from build123d import *

# Parameters (mm, degrees)
EXTRUDE_THIN1_DEPTH         = 393.7
F_1_4_CLEARANCE_HOLE1_D     = 6.7564
F_1_4_CLEARANCE_HOLE2_D     = 6.7564
F_1_4_CLEARANCE_HOLE2_DEPTH = 1.4478
CUT_EXTRUDE1_DEPTH          = 9.525


with BuildPart() as part:
    # Sketch1 → Extrude-Thin1 (new, symmetric)
    with BuildSketch(Plane(origin=(0, 0, 0), x_dir=(0, 0, -1), z_dir=(1, 0, 0))):
        with BuildLine():
            Line((-10.16, 25.4), (10.16, 25.4))
            ThreePointArc((10.16, 25.4), (11.956051224, 24.656051224), (12.7, 22.86))
            Line((12.7, 22.86), (12.7, -22.86))
            ThreePointArc((12.7, -22.86), (11.956051224, -24.656051224), (10.16, -25.4))
            Line((10.16, -25.4), (-10.16, -25.4))
            ThreePointArc((-10.16, -25.4), (-11.956051224, -24.656051224), (-12.7, -22.86))
            Line((-12.7, -22.86), (-12.7, 22.86))
            ThreePointArc((-12.7, 22.86), (-11.956051224, 24.656051224), (-10.16, 25.4))
        make_face()
        with BuildLine():
            Line((-10.16, 23.9522), (10.16, 23.9522))
            ThreePointArc((10.16, 23.9522), (10.932302026, 23.632302026), (11.2522, 22.86))
            Line((11.2522, 22.86), (11.2522, -22.86))
            ThreePointArc((11.2522, -22.86), (10.932302026, -23.632302026), (10.16, -23.9522))
            Line((10.16, -23.9522), (-10.16, -23.9522))
            ThreePointArc((-10.16, -23.9522), (-10.932302026, -23.632302026), (-11.2522, -22.86))
            Line((-11.2522, -22.86), (-11.2522, 22.86))
            ThreePointArc((-11.2522, 22.86), (-10.932302026, 23.632302026), (-10.16, 23.9522))
        make_face(mode=Mode.SUBTRACT)
    extrude(amount=EXTRUDE_THIN1_DEPTH, both=True)

    # 1/4 Clearance Hole1 (through all)
    with Locations(Plane(origin=(0, 0, -12.7), x_dir=(-1, 0, 0), z_dir=(0, 0, -1))):
        with Locations((-381, 15.875), (-381, -15.875), (-381, 0), (381, -15.875), (381, 0), (381, 15.875)):
            Hole(F_1_4_CLEARANCE_HOLE1_D / 2)

    # 1/4 Clearance Hole2
    with Locations(Plane(origin=(0, 0, -12.7), x_dir=(-1, 0, 0), z_dir=(0, 0, -1))):
        with Locations((-234.95, 15.875), (-234.95, 0), (-234.95, -15.875), (234.95, -15.875), (234.95, 0), (234.95, 15.875)):
            Hole(F_1_4_CLEARANCE_HOLE2_D / 2, depth=F_1_4_CLEARANCE_HOLE2_DEPTH)

    # Sketch6 → Cut-Extrude1 (cut)
    with BuildSketch(Plane(origin=(0, 0, -12.7), x_dir=(-1, 0, 0), z_dir=(0, 0, -1))):
        with BuildLine():
            Line((-120.65, -25.4), (-107.95, -25.4))
            Line((-107.95, -25.4), (-107.95, 15.875))
            ThreePointArc((-107.95, 15.875), (-108.87993597, 18.12006403), (-111.125, 19.05))
            Line((-111.125, 19.05), (-117.475, 19.05))
            ThreePointArc((-117.475, 19.05), (-119.72006403, 18.12006403), (-120.65, 15.875))
            Line((-120.65, 15.875), (-120.65, -25.4))
        make_face()
        with BuildLine():
            Line((-44.45, -25.4), (-31.75, -25.4))
            Line((-31.75, -25.4), (-31.75, 15.875))
            ThreePointArc((-31.75, 15.875), (-32.67993597, 18.12006403), (-34.925, 19.05))
            Line((-34.925, 19.05), (-41.275, 19.05))
            ThreePointArc((-41.275, 19.05), (-43.52006403, 18.12006403), (-44.45, 15.875))
            Line((-44.45, 15.875), (-44.45, -25.4))
        make_face()
        with BuildLine():
            Line((31.75, -25.4), (44.45, -25.4))
            Line((44.45, -25.4), (44.45, 15.875))
            ThreePointArc((44.45, 15.875), (43.52006403, 18.12006403), (41.275, 19.05))
            Line((41.275, 19.05), (34.925, 19.05))
            ThreePointArc((34.925, 19.05), (32.67993597, 18.12006403), (31.75, 15.875))
            Line((31.75, 15.875), (31.75, -25.4))
        make_face()
        with BuildLine():
            Line((107.95, -25.4), (120.65, -25.4))
            Line((120.65, -25.4), (120.65, 15.875))
            ThreePointArc((120.65, 15.875), (119.72006403, 18.12006403), (117.475, 19.05))
            Line((117.475, 19.05), (111.125, 19.05))
            ThreePointArc((111.125, 19.05), (108.87993597, 18.12006403), (107.95, 15.875))
            Line((107.95, 15.875), (107.95, -25.4))
        make_face()
    extrude(amount=-CUT_EXTRUDE1_DEPTH, mode=Mode.SUBTRACT)


solid = part.part
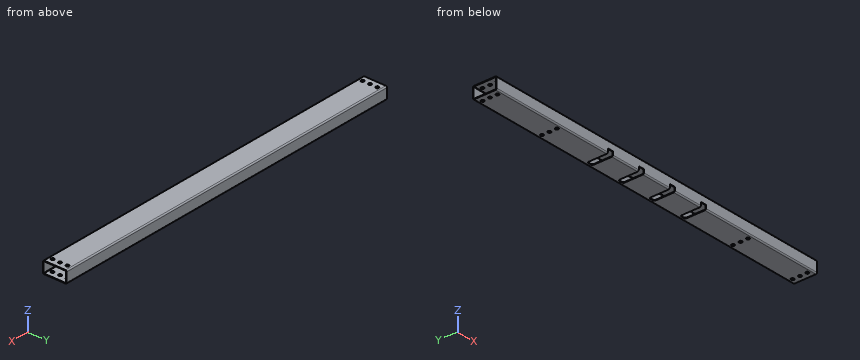
Here's how the part is built. I have some questions about the finished solid (model axes, mm). Give positions to 0.01 mm unless a question says otherwise; leave off trailing zeros. Loops run counter-clockwise (first coordinate to the right, second up) from the corner with the lowest first, then second, coordinate; pieces in that order, holes last. Notation, with made-up numbers: (28, 35) -> (81, 35) arc R34 ccw to (81, 68) -> close; hole circle Ø2 at (-19.75, 41). An arc over 180 degrees is marked (long way). Answer as a JSON object with one key per item and string values. Group by question number.
Item 1: Will these pins go through, and if not, where does the flat tip stop? pin 1 (1.2 mm diameter, centred on x = 112.5, y = -24.5, fed in from -Z) (3 decimals); pin 2 (0.7 mm diameter, centred on x = -115, z = -12, fed in from -Y).
Item 2: Imagine slicing it at A-A on z = 1.5. Write out the boundary of the cut face in (x, y).
Item 3: Imagine slicing it at B-B on x = -325. Write out the boundary of the cut face in (y, z), then the cut area to 3 significant figures.
Item 4: I need wall thicknesses on L1, parallel to Y at x = -62, z = -4.75; L2, parallel to Z at x = -310, y = 8.5; L3, parallel to Y at x = -381, z = 11.9. Which ranges of each line are inside material? Lowest first, please.
Answer list:
{
 "1": {"pin 1": "stops at z = -3.175", "pin 2": "stops at y = 19.05"},
 "2": {"outline": "(-393.7, -25.4) -> (393.7, -25.4) -> (393.7, -23.95) -> (-393.7, -23.95) -> close; (-393.7, 23.95) -> (393.7, 23.95) -> (393.7, 25.4) -> (-393.7, 25.4) -> close"},
 "3": {"outline": "(-25.4, -10.16) arc R2.54 ccw to (-22.86, -12.7) -> (22.86, -12.7) arc R2.54 ccw to (25.4, -10.16) -> (25.4, 10.16) arc R2.54 ccw to (22.86, 12.7) -> (-22.86, 12.7) arc R2.54 ccw to (-25.4, 10.16) -> close; hole (-23.95, -10.16) arc R1.09 ccw to (-22.86, -11.25) -> (22.86, -11.25) arc R1.09 ccw to (23.95, -10.16) -> (23.95, 10.16) arc R1.09 ccw to (22.86, 11.25) -> (-22.86, 11.25) arc R1.09 ccw to (-23.95, 10.16) -> close", "area": "208 mm2"},
 "4": {"L1": "y = -25.4 to -23.95, 23.95 to 25.4", "L2": "z = -12.7 to -11.25, 11.25 to 12.7", "L3": "y = -24.71 to -19.25, -12.5 to -3.38, 3.38 to 12.5, 19.25 to 24.71"}
}
